The model under review builds one solid part; all positions refer to its coordinate system, in mm. Coordinates: 2 decimals unless noted, no trailing zeros. Loops run counter-clockwise (first coordinate to the right, second up) from the corner with the lowest first, then second, coordinate; pieces in that order, holes last. Notation, with made-up numbers: M 52,14 L 66,14 A18 ccw 66,19 Z; hole C 88,18.25 d6. An arc over 180 degrees is marked long. Use CSV: the item, a comma, the result in double quotes. Start each with the question number.
1. Add section A-A, the plane y = 2.65. State how many separate pieces and enclosed holes the cut face has, then the cut area to 3 significant figures.
2. For L1, parallel to X at y = 4.7, z = -272; L2, parallel to Z at x = -202, y = 2.15; L3, parallel to Z at x = -52, y = 4.7, list the stretches that pass through material, from the lowest coordinate up.
3. Clearance check with flat-ended pins moving along their axes: P1, Ø1.8, axis at x = -36.5, y = 4.5, coming from the +Z side; P2, Ø3, axis at y = 1.5, z = -271, coming from the +X side. State where each tip first meets the part, or that it passes through.
4. Add section B-B, the plane x = 184. Write out the cut boundary in (y, z), then the cut area to 3 significant figures.
from build123d import *

# Parameters (mm, degrees)
SKETCH1_W           = 428
SKETCH1_H           = 538
BOSS_EXTRUDE1_DEPTH = 6
SKETCH2_W           = 40
SKETCH2_H           = 6
BOSS_EXTRUDE2_DEPTH = 6
SKETCH3_R           = 1.6
SKETCH3_R_2         = 2.1
CUT_EXTRUDE1_DEPTH  = 7


with BuildPart() as part:
    # Sketch1 → Boss-Extrude1 (new body)
    with BuildSketch(Plane(origin=(0, 0, 0), x_dir=(1, 0, 0), z_dir=(0, 1, 0))):
        Rectangle(SKETCH1_W, SKETCH1_H)
    extrude(amount=BOSS_EXTRUDE1_DEPTH)

    # Sketch2 → Boss-Extrude2 (add)
    with BuildSketch(Plane.XZ):
        with Locations((-100, 272)):
            Rectangle(SKETCH2_W, SKETCH2_H)
        with Locations((0, 272)):
            Rectangle(SKETCH2_W, SKETCH2_H)
        with Locations((100, 272)):
            Rectangle(SKETCH2_W, SKETCH2_H)
        with Locations((100, -272)):
            Rectangle(SKETCH2_W, SKETCH2_H)
        with Locations((0, -272)):
            Rectangle(SKETCH2_W, SKETCH2_H)
        with Locations((-100, -272)):
            Rectangle(SKETCH2_W, SKETCH2_H)
    extrude(amount=-BOSS_EXTRUDE2_DEPTH)

    # Sketch3 → Cut-Extrude1 (cut, through all)
    with BuildSketch(Plane.XZ):
        Polygon((204, -219.55), (207, -219.55), (207, -218.35), (214, -218.35), (214, -215.15), (207, -215.15), (207, -213.95), (204, -213.95), (204, -215.15), (199, -215.15), (199, -218.35), (204, -218.35), align=None)
        Polygon((-214, 229.35), (-214, 226.15), (-207, 226.15), (-207, 224.95), (-204, 224.95), (-204, 226.15), (-199, 226.15), (-199, 229.35), (-204, 229.35), (-204, 230.55), (-207, 230.55), (-207, 229.35), align=None)
        Polygon((-214, -215.15), (-214, -218.35), (-207, -218.35), (-207, -219.55), (-204, -219.55), (-204, -218.35), (-199, -218.35), (-199, -215.15), (-204, -215.15), (-204, -213.95), (-207, -213.95), (-207, -215.15), align=None)
        Polygon((207, 226.15), (214, 226.15), (214, 229.35), (207, 229.35), (207, 230.55), (204, 230.55), (204, 229.35), (199, 229.35), (199, 226.15), (204, 226.15), (204, 224.95), (207, 224.95), align=None)
        Polygon((151.6, 254), (151.6, 259), (152.8, 259), (152.8, 262), (151.6, 262), (151.6, 269), (148.4, 269), (148.4, 262), (147.2, 262), (147.2, 259), (148.4, 259), (148.4, 254), align=None)
        Polygon((51.6, 254), (51.6, 259), (52.8, 259), (52.8, 262), (51.6, 262), (51.6, 269), (48.4, 269), (48.4, 262), (47.2, 262), (47.2, 259), (48.4, 259), (48.4, 254), align=None)
        Polygon((-48.4, 254), (-48.4, 259), (-47.2, 259), (-47.2, 262), (-48.4, 262), (-48.4, 269), (-51.6, 269), (-51.6, 262), (-52.8, 262), (-52.8, 259), (-51.6, 259), (-51.6, 254), align=None)
        Polygon((-148.4, 254), (-148.4, 259), (-147.2, 259), (-147.2, 262), (-148.4, 262), (-148.4, 269), (-151.6, 269), (-151.6, 262), (-152.8, 262), (-152.8, 259), (-151.6, 259), (-151.6, 254), align=None)
        Polygon((-148.4, -254), (-151.6, -254), (-151.6, -259), (-152.8, -259), (-152.8, -262), (-151.6, -262), (-151.6, -269), (-148.4, -269), (-148.4, -262), (-147.2, -262), (-147.2, -259), (-148.4, -259), align=None)
        Polygon((-48.4, -254), (-51.6, -254), (-51.6, -259), (-52.8, -259), (-52.8, -262), (-51.6, -262), (-51.6, -269), (-48.4, -269), (-48.4, -262), (-47.2, -262), (-47.2, -259), (-48.4, -259), align=None)
        Polygon((51.6, -254), (48.4, -254), (48.4, -259), (47.2, -259), (47.2, -262), (48.4, -262), (48.4, -269), (51.6, -269), (51.6, -262), (52.8, -262), (52.8, -259), (51.6, -259), align=None)
        Polygon((151.6, -254), (148.4, -254), (148.4, -259), (147.2, -259), (147.2, -262), (148.4, -262), (148.4, -269), (151.6, -269), (151.6, -262), (152.8, -262), (152.8, -259), (151.6, -259), align=None)
        with Locations((-100, -272)):
            Circle(SKETCH3_R)
        with Locations((0, -272)):
            Circle(SKETCH3_R)
        with Locations((100, -272)):
            Circle(SKETCH3_R)
        with Locations((202, 257)):
            Circle(SKETCH3_R_2)
        with Locations((-202, 257)):
            Circle(SKETCH3_R_2)
    extrude(amount=-CUT_EXTRUDE1_DEPTH, mode=Mode.SUBTRACT)


solid = part.part
Computed:
1,separate pieces,"1"
1,enclosed holes,"5"
1,area,"231,000 mm^2"
2,L1,"x = -120 to -101.6, -98.4 to -80, -20 to -1.6, 1.6 to 20, 80 to 98.4, 101.6 to 120"
2,L2,"z = -269 to -218.35, -215.15 to 226.15, 229.35 to 254.9, 259.1 to 269"
2,L3,"z = -269 to -262, -259 to 259, 262 to 269"
3,P1,"stops at z = 269"
3,P2,"stops at x = 120"
4,outline,"M 0,-269 L 6,-269 L 6,269 L 0,269 Z"
4,area,"3,230 mm^2"
